Input: part model. Units: mm. Frame: model coordinates. Face numbers are marked on the shaded views. Coordinates: 2 decimals unless noted, no trailing zeros. Loops run counter-clockwise (first coordinate to the right, second up) from the corner with the lowest first, then second, coordinate; pieces in that order, holes last. Notation, with made-up numbers: (-28.75, 9) - (17.25, 9) arc R20 ccw to (17.25, 25) - close; hole circle Ø3 at (-4.5, 69.5). An arc over 180 degrees is marked (long way). Use a Markdown table: item, result. Add a question column.
1. Section query B-B on z = 12.25. Return the cut outline in (x, y).
2. Draft query along X for the marked faces 1, 2, 3 and 4. Return one class per face: released by +X, released by -X, zero draft, split by the parting line, or undercut.
3. Section query D-D on z = 2.75. Return the cut outline in (x, y), then the cut area to 3 significant figures.
4. Ray query, L1, parallel to Y at x = 10, z = 5.5; L2, parallel to Y at x = 10, z = 15.25; L3, parallel to X at y = 11, z = 14.75. Return the intervals inside material, ascending. Write a range as [from, to].
5. Section query A-A on x = 10. Return the cut outline in (y, z), then the cut area to 3 significant figures.
6. Section query C-C on z = 9.5. Return the cut outline in (x, y), then the cut area to 3 significant figures.
7. Contact query for a flat-ended pin moving along its axis: P1, Ø3, axis at x = 10.5, y = 13, coming from the -Z side. Output: stop coordinate, or through.
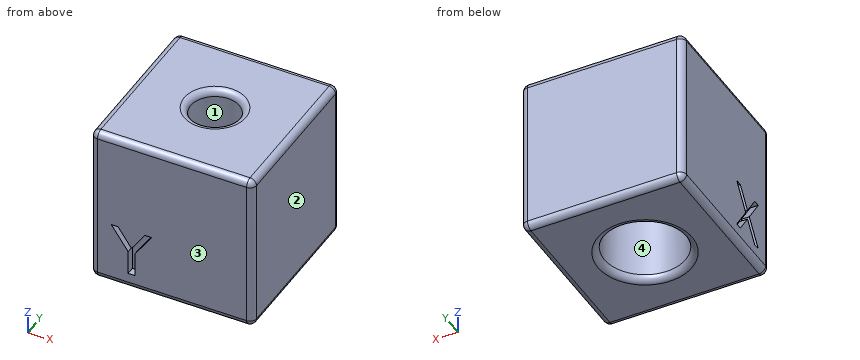
```python
from build123d import *

# Parameters (mm, degrees)
SKETCH_W        = 20
SKETCH_H        = 20
PAD_DEPTH       = 20
POCKET_DEPTH    = 1
POCKET001_DEPTH = 1
SKETCH004_R     = 5
HOLE_DEPTH      = 10
HOLE_TIPS_R     = 5
SKETCH005_R     = 3
HOLE001_DEPTH   = 10
HOLE001_TIPS_R  = 3
FILLET_R        = 0.8
FILLET001_R     = 0.8


with BuildPart() as part:
    # Sketch → Pad (new body)
    with BuildSketch(Plane.XY):
        with Locations((10, 10)):
            Rectangle(SKETCH_W, SKETCH_H)
    extrude(amount=PAD_DEPTH)

    # Sketch002 → Pocket (cut)
    with BuildSketch(Plane.YZ):
        Polygon((7.5, 8), (6.666667, 8), (5, 5.6), (3.333333, 8), (2.5, 8), (4.583333, 5), (2.5, 2), (3.333333, 2), (5, 4.4), (6.666667, 2), (7.5, 2), (5.416667, 5), align=None)
    extrude(amount=POCKET_DEPTH, mode=Mode.SUBTRACT)

    # Sketch003 → Pocket001 (cut)
    with BuildSketch(Plane.XZ):
        Polygon((2.5, 8), (3.333333, 8), (5, 5.6), (6.666667, 8), (7.5, 8), (5.416667, 5), (5.416667, 2), (4.583333, 2), (4.583333, 5), align=None)
    extrude(amount=-POCKET001_DEPTH, mode=Mode.SUBTRACT)

    # Sketch004 → Hole (cut)
    with BuildSketch(Plane.XY):
        with Locations((10, 10)):
            Circle(SKETCH004_R)
    extrude(amount=HOLE_DEPTH, mode=Mode.SUBTRACT)

    # Hole tips → Hole tip 1 section 0
    with BuildSketch(Plane.XY.offset(10), mode=Mode.PRIVATE) as hole_tip_1_s0:
        with Locations((10, 10)):
            Circle(HOLE_TIPS_R)
    loft([hole_tip_1_s0.sketch, Vertex(10, 10, 13.004303)], mode=Mode.SUBTRACT)

    # Sketch005 (on DatumPlane) → Hole001 (cut)
    with BuildSketch(Plane.XY.offset(20)):
        with Locations((10, 10)):
            Circle(SKETCH005_R)
    extrude(amount=-HOLE001_DEPTH, mode=Mode.SUBTRACT)

    # Hole001 tips → Hole001 tip 1 section 0
    with BuildSketch(Plane.XY.offset(10), mode=Mode.PRIVATE) as hole001_tip_1_s0:
        with Locations((10, 10)):
            Circle(HOLE001_TIPS_R)
    loft([hole001_tip_1_s0.sketch, Vertex(10, 10, 8.197418)], mode=Mode.SUBTRACT)

    # Fillet
    fillet_edges = [part.edges().sort_by_distance(p)[0] for p in [
        (0, 0, 10),
        (0, 10, 20),
        (0, 20, 10),
        (10, 20, 20),
        (0, 10, 0),
        (10, 20, 0),
        (20, 20, 10),
        (20, 10, 0),
        (20, 0, 10),
        (10, 0, 0),
        (20, 10, 20),
        (10, 0, 20),
    ]]
    fillet(fillet_edges, radius=FILLET_R)

    # Fillet001
    fillet001_edges = [part.edges().sort_by_distance(p)[0] for p in [
        (7, 10, 20),
        (15, 10, 0),
    ]]
    fillet(fillet001_edges, radius=FILLET001_R)


solid = part.part
```
Resolved:
| question | item | result |
|---|---|---|
| 1 | outline | (0, 0.8) arc R0.8 ccw to (0.8, 0) - (19.2, 0) arc R0.8 ccw to (20, 0.8) - (20, 19.2) arc R0.8 ccw to (19.2, 20) - (0.8, 20) arc R0.8 ccw to (0, 19.2) - close; hole circle Ø6 at (10, 10) |
| 2 | face 1 | undercut |
| 2 | face 2 | released by +X |
| 2 | face 3 | zero draft |
| 2 | face 4 | undercut |
| 3 | outline | (0, 0.8) arc R0.8 ccw to (0.8, 0) - (4.58, 0) - (4.58, 1) - (5.42, 1) - (5.42, 0) - (19.2, 0) arc R0.8 ccw to (20, 0.8) - (20, 19.2) arc R0.8 ccw to (19.2, 20) - (0.8, 20) arc R0.8 ccw to (0, 19.2) - (0, 6.98) - (1, 6.98) - (1, 6.15) - (0, 6.15) - (0, 3.85) - (1, 3.85) - (1, 3.02) - (0, 3.02) - close; hole circle Ø10 at (10, 10) |
| 3 | area | 318 mm² |
| 4 | L1 | [0, 5], [15, 20] |
| 4 | L2 | [0, 7], [13, 20] |
| 4 | L3 | [0, 7.17], [12.83, 20] |
| 5 | outline | (0, 0.8) arc R0.8 ccw to (0.8, 0) - (4.2, 0) arc R0.8 ccw to (5, 0.8) - (5, 10) - (7, 11.2) - (7, 19.2) arc R0.8 ccw to (6.2, 20) - (0.8, 20) arc R0.8 ccw to (0, 19.2) - close; (13, 11.2) - (15, 10) - (15, 0.8) arc R0.8 ccw to (15.8, 0) - (19.2, 0) arc R0.8 ccw to (20, 0.8) - (20, 19.2) arc R0.8 ccw to (19.2, 20) - (13.8, 20) arc R0.8 ccw to (13, 19.2) - close |
| 5 | area | 236 mm² |
| 6 | outline | (0, 0.8) arc R0.8 ccw to (0.8, 0) - (19.2, 0) arc R0.8 ccw to (20, 0.8) - (20, 19.2) arc R0.8 ccw to (19.2, 20) - (0.8, 20) arc R0.8 ccw to (0, 19.2) - close; hole circle Ø10 at (10, 10) |
| 6 | area | 321 mm² |
| 7 | P1 | z = 10.28 |
